from build123d import *

# Parameters (mm, degrees)
SKETCH1_W           = 96
SKETCH1_H           = 90
BOSS_EXTRUDE1_DEPTH = 5
SKETCH2_R           = 1.5
CUT_EXTRUDE1_DEPTH  = 6
SKETCH3_R           = 1.5
CUT_EXTRUDE2_DEPTH  = 6


with BuildPart() as part:
    # Sketch1 → Boss-Extrude1 (new body)
    with BuildSketch(Plane.XY):
        Rectangle(SKETCH1_W, SKETCH1_H)
    extrude(amount=BOSS_EXTRUDE1_DEPTH)

    # Sketch2 → Cut-Extrude1 (cut, through all)
    with BuildSketch(Plane.XY.offset(5)):
        with Locations((45.5, 11.5)):
            Circle(SKETCH2_R)
        with Locations((45.5, -23.5)):
            Circle(SKETCH2_R)
    extrude(amount=-CUT_EXTRUDE1_DEPTH, mode=Mode.SUBTRACT)

    # Sketch3 → Cut-Extrude2 (cut, through all)
    with BuildSketch(Plane.XY.offset(5)):
        with Locations((-44, 25)):
            Circle(SKETCH3_R)
        with Locations((-44, -25)):
            Circle(SKETCH3_R)
    extrude(amount=-CUT_EXTRUDE2_DEPTH, mode=Mode.SUBTRACT)


solid = part.part
Here's how the part is built. I have some questions about the finished solid (model axes, mm). Round coordinates to 2 decimals unless told otherwise and drop trailing zeros. Loops run counter-clockwise (first coordinate to the right, second up) from the corner with the lowest first, then second, coordinate; pieces in that order, holes last. Notation, with made-up numbers: (28.5, -18.5) - (34.5, -18.5) arc R22 ccw to (34.5, 9.5) - close; hole circle Ø9 at (51.5, 52). An arc over 180 degrees is marked (long way). One line per question, with ' | ' between items. Start each with the question number.
Q1. Please list where these lines run through material, in increasing order: line 1 (Y direction, x = 45.5, z = 3.6); line 2 (Y direction, x = -44, z = 3); line 3 (X direction, y = 24, z = 3.8). Write a range as [from, to].
Q2. We'd pull the mould along Y, two halves only. Please class faces 1 (the cylindrical face through (-45.11, -23.99, 2.54)), 2 (the flat face through (-1, 1, 5)), 3 (the flat face through (-1, 45, 2)): +Y half, -Y half, draft (parallel to the pull), parting line (faces both ways), or undercut.
Q3. I want a section at A-A (y = 11.5). Write out the boundary of the cut face in (x, z), then the cut area to 3 significant figures.
Q4. I want a section at B-B (x = 45.5). Write out the boundary of the cut face in (y, z), then the cut area to 3 significant figures.
Response values:
1) line 1: y = [-45, -25], [-22, 10], [13, 45] | line 2: y = [-45, -26.5], [-23.5, 23.5], [26.5, 45] | line 3: x = [-48, -45.12], [-42.88, 48]
2) face 1: undercut | face 2: draft | face 3: +Y half
3) outline: (-48, 0) - (44, 0) - (44, 5) - (-48, 5) - close; (47, 0) - (48, 0) - (48, 5) - (47, 5) - close | area: 465 mm²
4) outline: (-45, 0) - (-25, 0) - (-25, 5) - (-45, 5) - close; (-22, 0) - (10, 0) - (10, 5) - (-22, 5) - close; (13, 0) - (45, 0) - (45, 5) - (13, 5) - close | area: 420 mm²
